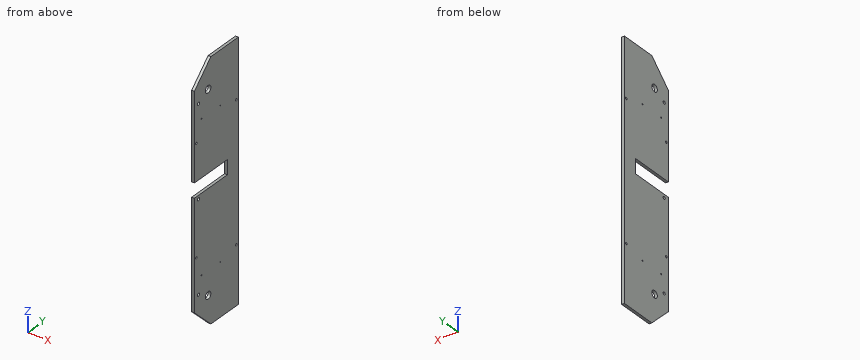
Autodesk Inventor part; units mm, degrees
ref_plane "YZ Plane" through (0, 0, 0) normal (1, 0, 0) x (0, 1, 0)
ref_plane "XZ Plane" through (0, 0, 0) normal (0, 1, 0) x (-1, 0, 0)
ref_plane "XY Plane" through (0, 0, 0) normal (0, 0, 1) x (1, 0, 0)
sketch "Sketch1" plane through (0, 0, 0) normal (1, 0, 0) x (0, 1, 0)
  line L0 (0, 0) -> (101.6, 0)
  line L1 (101.6, 0) -> (101.6, -444.5)
  line L2 (101.6, -444.5) -> (0, -444.5)
  line L3 (0, -444.5) -> (0, 0)
  circle A0 centre (31.75, -50.8) radius 6.3627
  circle A1 centre (31.75, -393.7) radius 6.3627
  circle A2 centre (86.2838, -165.5318) radius 1.5875
  circle A3 centre (70.2818, -165.5318) radius 1.5875
  circle A4 centre (15.3162, -278.9682) radius 1.5875
  circle A5 centre (31.3182, -278.9682) radius 1.5875
  dimension "d0" = 101.6
  dimension "d1" = 444.5
  dimension "d2" = 12.7254
  dimension "d3" = 31.75
  dimension "d4" = 50.8
  dimension "d5" = 50.8
  dimension "d22" = 165.5318
  dimension "d23" = 3.175
  dimension "d24" = 15.3162
  dimension "d25" = 3.175
  dimension "d26" = 16.002
  dimension "d27" = 165.5318
  dimension "d28" = 3.175
  dimension "d29" = 15.3162
  dimension "d30" = 165.5318
  dimension "d31" = 3.175
  dimension "d32" = 16.002
  dimension "d33" = 165.5318
extrude "Extrusion1" add sketch "Sketch1" along normal blind 4.7625 contours L0 L1 L2 L3 | A2 | A3 | A4 | A5
chamfer "Chamfer1" distance 38.1 angle 45 1 edges at (2.3813, 0, 0)
chamfer "Chamfer2" distance 38.1 angle 45 1 edges at (2.3813, 0, -444.5)
sketch "Sketch6" plane through (4.7625, 0, 0) normal (1, 0, 0) x (0, 0, -1)
  line L0 (444.5, 38.1) -> (406.4, 0)
  line L1 (444.5, 38.1) -> (444.5, 101.6)
  line L2 (444.5, 101.6) -> (0, 101.6)
  line L3 (0, 101.6) -> (0, 38.1)
  line L4 (38.1, 0) -> (0, 38.1)
  line L5 (38.1, 0) -> (406.4, 0)
  circle A0 centre (393.7, 31.75) radius 6.3627
  circle A1 centre (50.8, 31.75) radius 6.3627
  point P0 (0, 0)
  point P1 (92.075, 59.69)
  point P2 (92.075, 16.51)
  point P3 (352.425, 59.69)
  point P4 (352.425, 16.51)
  dimension "d80" = 43.18
  dimension "d83" = 16.51
  dimension "d86" = 43.18
  dimension "d115" = 92.075
  dimension "d116" = 92.075
  dimension "d117" = 16.51
  dimension "d118" = 92.075
  dimension "d119" = 92.075
hole "Hole1" at (4.7625, 59.69, -92.075) at (4.7625, 16.51, -92.075) at (4.7625, 59.69, -352.425) at (4.7625, 16.51, -352.425) direction (-1, 0, 0) diameter 2.032 end through all
sketch "Sketch7" plane through (4.7625, 0, 0) normal (1, 0, 0) x (0, 0, -1)
  circle A0 centre (352.425, 59.69) radius 1.016
  circle A1 centre (92.075, 59.69) radius 1.016
  circle A2 centre (92.075, 16.51) radius 1.016
  circle A3 centre (352.425, 16.51) radius 1.016
  line L0 (444.5, 38.1) -> (406.4, 0)
  line L1 (444.5, 38.1) -> (444.5, 101.6)
  line L2 (444.5, 101.6) -> (0, 101.6)
  line L3 (0, 101.6) -> (0, 38.1)
  line L4 (38.1, 0) -> (0, 38.1)
  line L5 (38.1, 0) -> (406.4, 0)
  circle A4 centre (393.7, 31.75) radius 6.3627
  circle A5 centre (50.8, 31.75) radius 6.3627
  point P0 (0, 0)
  point P1 (101.6, 97.155)
  point P2 (342.9, 97.155)
  point P3 (127, 4.445)
  point P4 (317.5, 4.445)
  dimension "d95" = 4.445
  dimension "d96" = 4.445
  dimension "d97" = 4.445
  dimension "d98" = 4.445
  dimension "d99" = 101.6
  dimension "d100" = 101.6
  dimension "d101" = 127
  dimension "d102" = 127
hole "Hole2" at (4.7625, 97.155, -101.6) at (4.7625, 97.155, -342.9) at (4.7625, 4.445, -127) at (4.7625, 4.445, -317.5) direction (-1, 0, 0) diameter 3.81 depth 25.4 tip angle 118
sketch "Sketch8" plane through (4.7625, 0, 0) normal (1, 0, 0) x (0, 0, -1)
  line L0 (406.4, 0) -> (38.1, 0)
  line L1 (190.5, 0) -> (215.9, 0)
  line L2 (215.9, 0) -> (215.9, 76.2)
  line L3 (215.9, 76.2) -> (190.5, 76.2)
  line L4 (190.5, 76.2) -> (190.5, 0)
  line L5 (0, 101.6) -> (0, 38.1)
  point P0 (0, 0)
  dimension "d112" = 25.4
  dimension "d113" = 190.5
  dimension "d114" = 76.2
extrude "Extrusion6" cut sketch "Sketch8" against normal through all
sketch "Sketch9" plane through (4.7625, 0, 0) normal (1, 0, 0) x (0, 0, -1)
  line L0 (38.1, 0) -> (190.5, 0)
  line L1 (0, 101.6) -> (0, 38.1)
  line L2 (444.5, 38.1) -> (444.5, 101.6)
  point P0 (0, 0)
  point P1 (63.5, 9.525)
  point P2 (222.25, 9.525)
  point P3 (381, 9.525)
  dimension "d120" = 9.525
  dimension "d121" = 63.5
  dimension "d122" = 63.5
  dimension "d123" = 317.5
  dimension "d124" = 158.75
hole "Hole3" at (4.7625, 9.525, -63.5) at (4.7625, 9.525, -222.25) at (4.7625, 9.525, -381) direction (-1, 0, 0) diameter 5.08 depth 19.05 tip angle 118
properties part number "DriveTrain3.0" material "Aluminum 6061"
Verification items for the finished model (mm, model axes). Give positions to 0.01 mm unless a question says otherwise; leave off trailing zeros. Loops run counter-clockwise (first coordinate to the right, second up) from the corner with the lowest first, then second, coordinate; pieces in that order, holes last. Notation, with made-up numbers: M -2,-6.5 L 32,-6.5 A32 cw 32,31.5 Z; hole C 88.25,54.25 d1. An arc over 180 degrees is marked long. One line per question, with ' | ' between items.
Item 1: Thickness scan on line 1 (Y direction, x = 1.85, z = -343); line 2 (Z direction, x = 1.85, y = 76); line 3 (Z direction, x = 0.2, y = 31). Record the ranges inside material, lowest first. Write a range as [from, to].
Completed:
line 1: y = [0, 95.25], [99.06, 101.6] | line 2: z = [-444.5, -215.9], [-190.5, 0] | line 3: z = [-437.4, -400.02], [-387.38, -215.9], [-190.5, -57.12], [-44.48, -7.1]
Item 2: Depth check by flat-ended pin: P1, Ø3.5, axis at y = 97.155, z = -342.9, coming from the -X side. Enter the tip coordinate at first touch or a pass-through.
Completed:
P1: passes through
Item 3: Section check A-A, the plane y = 31.75. Record the cut outline in (x, z).
Completed:
outline: M 0,-438.15 L 4.76,-438.15 L 4.76,-400.06 L 0,-400.06 Z; M 0,-387.34 L 4.76,-387.34 L 4.76,-215.9 L 0,-215.9 Z; M 0,-190.5 L 4.76,-190.5 L 4.76,-57.16 L 0,-57.16 Z; M 0,-44.44 L 4.76,-44.44 L 4.76,-6.35 L 0,-6.35 Z
Item 4: Section check C-C, the plane y = 65.5. Record the cut outline in (x, z).
Completed:
outline: M 0,-444.5 L 4.76,-444.5 L 4.76,-215.9 L 0,-215.9 Z; M 0,-190.5 L 4.76,-190.5 L 4.76,0 L 0,0 Z
Item 5: Section check B-B, the plane z = -393.7. Record the cut outline in (x, y), plus the area to 3 significant figures.
Completed:
outline: M 0,0 L 4.76,0 L 4.76,25.39 L 0,25.39 Z; M 0,38.11 L 4.76,38.11 L 4.76,101.6 L 0,101.6 Z | area: 423 mm^2
Item 6: Section check D-D, the plane x = 3.5. State how many separate pieces and enclosed holes the cut face has, plus the area to 3 significant figures.
Completed:
separate pieces: 1 | enclosed holes: 13 | area: 41,400 mm^2
